Print and shaded views of the part. All mm, measured from the part's lowest x, y and z. Coordinates: 2 decimals unless noted, no trailing zeros. Order: outer loops, then holes, each group sorted by start corner. A loop starts at its lowest first (then second) coordinate and runs counter-clockwise, first axis right, second up. Notation, with made-up numbers: M 22,-36 L 79,-36 A23 ccw 79,1 Z; hole C 34.5,6 d9. An arc over 180 degrees is marked long. Return JSON: item names as keys, results as strings.
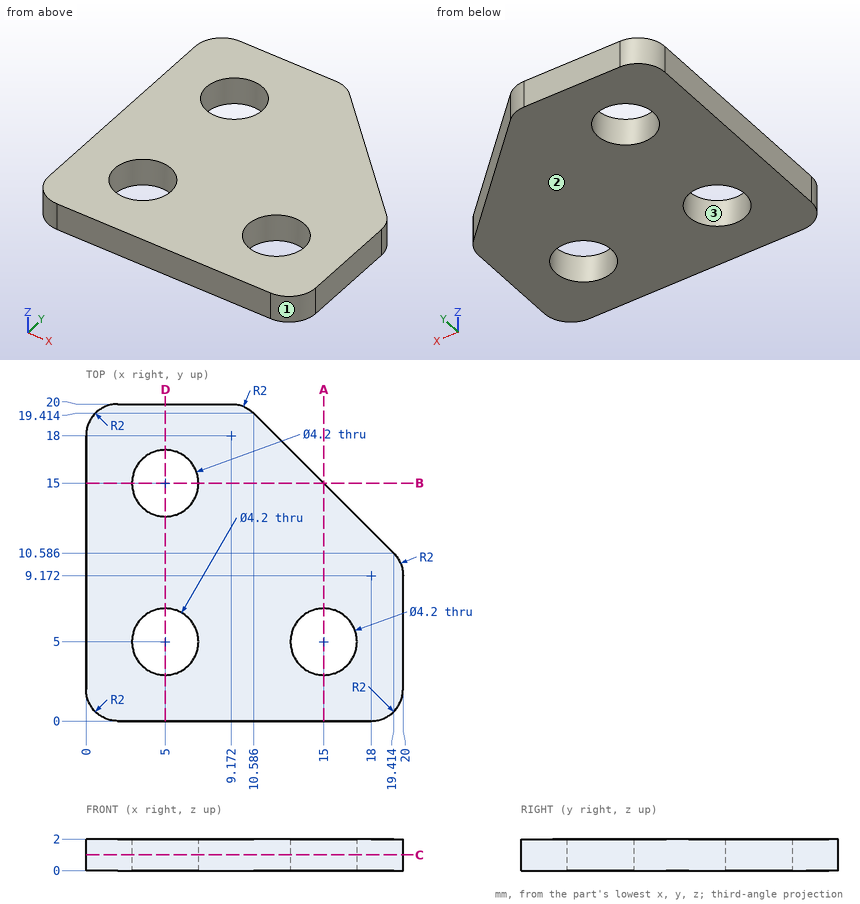
Item 1: Pull direction Y, two halves, no side cores. Call the marked faces 1, 2 and 3: +Y half, -Y half, draft (parallel to the pull), parting line (faces both ways), or undercut.
Check result:
{"face 1": "-Y half", "face 2": "draft", "face 3": "undercut"}
Item 2: Wall check: line 1 (Y direction, x = 5, z = 0.65); line 2 (Y direction, x = 4.5, z = 1.95); line 3 (Y direction, x = 16, z = 0.95) (1 decimal). Give the ranges that are in metal, low to high.
Check result:
{"line 1": "y = 0 to 2.9, 7.1 to 12.9, 17.1 to 20", "line 2": "y = 0 to 2.96, 7.04 to 12.96, 17.04 to 20", "line 3": "y = 0 to 3.2, 6.8 to 14"}
Item 3: Saw through at A-A (x = 15). Write the cut outline in (y, z), and give its area (3 significant figures).
Check result:
{"outline": "M 0,0 L 2.9,0 L 2.9,2 L 0,2 Z; M 7.1,0 L 15,0 L 15,2 L 7.1,2 Z", "area": "21.6 mm2"}
Item 4: Saw through at C-C (z = 1). Write the cut outline in (x, y) (1 decimal), and give its area (3 significant figures).
Check result:
{"outline": "M 0,2 A2 ccw 2,0 L 18,0 A2 ccw 20,2 L 20,9.2 A2 ccw 19.4,10.6 L 10.6,19.4 A2 ccw 9.2,20 L 2,20 A2 ccw 0,18 Z; hole C 5,5 d4.2; hole C 5,15 d4.2; hole C 15,5 d4.2", "area": "306 mm2"}
Item 5: Saw through at D-D (x = 5). Write the cut outline in (y, z).
Check result:
{"outline": "M 0,0 L 2.9,0 L 2.9,2 L 0,2 Z; M 7.1,0 L 12.9,0 L 12.9,2 L 7.1,2 Z; M 17.1,0 L 20,0 L 20,2 L 17.1,2 Z"}
Item 6: Drop a flat-ended pin along its axis: pin 1 Ø5.5 at (x, y) = (5, 15) entering from +Z. Give the stop position or say it passes through.
Check result:
{"pin 1": "stops at z = 2"}
